```python
from build123d import *

# Parameters (mm, degrees)
SKETCH_1_R      = 4.5
SKETCH_1_R_2    = 2.5
EXTRUDE_1_DEPTH = 5
SKETCH_2_R      = 3
EXTRUDE_2_DEPTH = 28
EXTRUDE_3_DEPTH = 4
SKETCH_5_R      = 3
EXTRUDE_4_DEPTH = 5.5
EXTRUDE_6_DEPTH = 5
SKETCH_7_R      = 1.6
EXTRUDE_7_DEPTH = 1.4


with BuildPart() as part:
    # 草图1 → 凸台-拉伸1 (new body)
    with BuildSketch(Plane(origin=(0, 0, 0), x_dir=(0, 0, -1), z_dir=(1, 0, 0))):
        with BuildLine():
            Line((31.1, -15.85), (-21.1, -15.85))
            ThreePointArc((-21.1, -15.85), (-28.171067812, -12.921067812), (-31.1, -5.85))
            Line((-31.1, -5.85), (-31.1, 5.85))
            ThreePointArc((-31.1, 5.85), (-28.171067812, 12.921067812), (-21.1, 15.85))
            Line((-21.1, 15.85), (31.1, 15.85))
            Line((31.1, 15.85), (31.1, -15.85))
        make_face()
        with Locations((-11.1, 0)):
            Circle(SKETCH_1_R, mode=Mode.SUBTRACT)
        with Locations((13.4, 0)):
            Circle(SKETCH_1_R_2, mode=Mode.SUBTRACT)
    extrude(amount=EXTRUDE_1_DEPTH)

    # 草图2 → 凸台-拉伸2 (add)
    with BuildSketch(Plane(origin=(5, 0, 0), x_dir=(0, 0, -1), z_dir=(1, 0, 0))):
        with Locations((-28.1, 0)):
            Circle(SKETCH_2_R)
        with Locations((4.1, 11.85)):
            Circle(SKETCH_2_R)
        with Locations((4.1, -11.85)):
            Circle(SKETCH_2_R)
    extrude(amount=EXTRUDE_2_DEPTH)

    # 草图3 → 凸台-拉伸3 (add)
    with BuildSketch(Plane(origin=(33, 0, 0), x_dir=(0, 0, -1), z_dir=(1, 0, 0))):
        with BuildLine():
            Line((8.9, 15.85), (-21.1, 15.85))
            ThreePointArc((-21.1, 15.85), (-28.171067812, 12.921067812), (-31.1, 5.85))
            Line((-31.1, 5.85), (-31.1, 0))
            Line((-31.1, 0), (-31.1, -5.85))
            ThreePointArc((-31.1, -5.85), (-28.171067812, -12.921067812), (-21.1, -15.85))
            Line((-21.1, -15.85), (8.9, -15.85))
            Line((8.9, -15.85), (8.9, 15.85))
        make_face()
    extrude(amount=EXTRUDE_3_DEPTH)

    # 草图5 → 凸台-拉伸4 (add)
    with BuildSketch(Plane.ZY):
        with Locations((-27.1, 11.85)):
            Circle(SKETCH_5_R)
        with Locations((-27.1, -11.978090594)):
            Circle(SKETCH_5_R)
        with Locations((13.9, 11.85)):
            Circle(SKETCH_5_R)
        with Locations((13.9, -11.978090594)):
            Circle(SKETCH_5_R)
    extrude(amount=EXTRUDE_4_DEPTH)

    # 草图6 → 凸台-拉伸6 (add)
    with BuildSketch(Plane.ZY.offset(5.5)):
        with BuildLine():
            Line((15.255672946, -15.85), (-31.1, -15.85))
            Line((-31.1, -15.85), (-31.1, 15.85))
            Line((-31.1, 15.85), (15.255672946, 15.85))
            ThreePointArc((15.255672946, 15.85), (17.376993289, 14.971320344), (18.255672946, 12.85))
            Line((18.255672946, 12.85), (18.255672946, 9.183659284))
            ThreePointArc((18.255672946, 9.183659284), (17.376993289, 7.062338941), (15.255672946, 6.183659284))
            Line((15.255672946, 6.183659284), (8.696116264, 6.183659284))
            ThreePointArc((8.696116264, 6.183659284), (6.574795921, 5.304979628), (5.696116264, 3.183659284))
            Line((5.696116264, 3.183659284), (5.696116264, -3.183659284))
            ThreePointArc((5.696116264, -3.183659284), (6.574795921, -5.304979628), (8.696116264, -6.183659284))
            Line((8.696116264, -6.183659284), (15.255672946, -6.183659284))
            ThreePointArc((15.255672946, -6.183659284), (17.376993289, -7.062338941), (18.255672946, -9.183659284))
            Line((18.255672946, -9.183659284), (18.255672946, -12.85))
            ThreePointArc((18.255672946, -12.85), (17.376993289, -14.971320344), (15.255672946, -15.85))
        make_face()
    extrude(amount=EXTRUDE_6_DEPTH)

    # 草图7 → 凸台-拉伸7 (add)
    with BuildSketch(Plane.XZ.offset(15.85)):
        with Locations((2.5, 10.7)):
            Circle(SKETCH_7_R)
        with Locations((2.5, -23.1)):
            Circle(SKETCH_7_R)
    extrude(amount=EXTRUDE_7_DEPTH)


solid = part.part
```
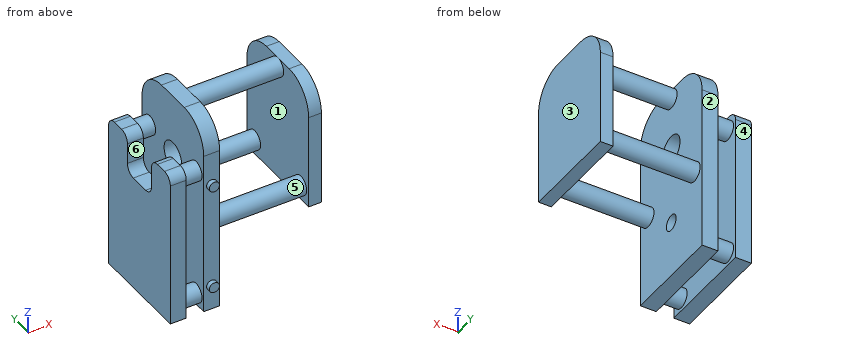
Here's how the part is built. I have some questions about the finished solid (model axes, mm). Face numbers are marked on the shaded views. A direction names the side the tool comes from. Coordinates: 2 decimals unless noted, no trailing zeros. Order: outer loops, then holes, each group sorted by start corner. A loop starts at its lowest first (then second) coordinate and runs counter-clockwise, first axis right, second up. Notation, with made-up numbers: (-26.5, 84) - (10.5, 84) arc R21 ccw to (10.5, 119) - close; hole circle Ø6 at (49.5, 66). An arc over 180 degrees is marked (long way). One line per question, with ' | ' between items.
(1) If I drill on L1, parallel to X at y = 9.5, z = 8; L2, parallel to X at y = -9.5, z = 22.5; L3, parallel to Y at x = 2, z = 11, over which ranges is the centre line in solid material (lowest first)?
Report:
L1: x = -10.5 to -5.5, 0 to 5, 33 to 37 | L2: x = 0 to 5, 33 to 37 | L3: y = -17.25 to -4.5, 4.5 to 15.85
(2) Suppose I cut it at B-B on z = -23.1. List the corners of the cut face in (x, y) for me.
Report:
outline: (-10.5, -15.85) - (-5.5, -15.85) - (-5.5, 15.85) - (-10.5, 15.85) - close; (0, -15.85) - (0.9, -15.85) - (0.9, -17.25) - (4.1, -17.25) - (4.1, -15.85) - (5, -15.85) - (5, 15.85) - (0, 15.85) - close
(3) For the marked faces 1 and 2, which set-ups out of +Z, -Z, +X, -X, +Y, -Y let a thin tool reach every point of the face, with its end or its side?
Report:
face 1: none | face 2: +Z, -Z, +X, -X, +Y
(4) Suppose I cut it at C-C on x = 2.5. List the corners of the cut face in (y, z) for me.
Report:
outline: (-17.25, -24.7) - (-15.85, -24.7) - (-15.85, -31.1) - (15.85, -31.1) - (15.85, 21.1) arc R10 ccw to (5.85, 31.1) - (-5.85, 31.1) arc R10 ccw to (-15.85, 21.1) - (-15.85, 12.3) - (-17.25, 12.3) - (-17.25, 9.1) - (-15.85, 9.1) - (-15.85, -21.5) - (-17.25, -21.5) - close; hole circle Ø9 at (0, 11.1); hole circle Ø5 at (0, -13.4)
(5) Suppose I cut it at A-A on z = -4.1. List the corners of the cut face in (x, y) for me, and give its area (3 significant figures).
Report:
outline: (-10.5, -15.85) - (-5.5, -15.85) - (-5.5, 15.85) - (-10.5, 15.85) - close; (0, -15.85) - (5, -15.85) - (5, -14.85) - (33, -14.85) - (33, -15.85) - (37, -15.85) - (37, 15.85) - (33, 15.85) - (33, 14.85) - (5, 14.85) - (5, 15.85) - (0, 15.85) - close; hole (5, -8.85) - (33, -8.85) - (33, 8.85) - (5, 8.85) - close | area: 780 mm2
(6) Will these pins go through, and if not, where does the flat tip stop? pin 1 (1.5 mm diameter, centred on x = -3, y = 2.5, fed in from +Z); pin 2 (3 mm diameter, centred on x = -7.5, y = 11, fed in from +Z); pin 3 (3 mm diameter, centred on y = 0, z = -13.4, fed in from +X); pin 4 (11.5 mm diameter, centred on y = 0, z = 11.1, fed in from -X).
Report:
pin 1: passes through | pin 2: stops at z = 18.26 | pin 3: stops at x = -5.5 | pin 4: stops at x = -10.5
(7) Suppose I cut it at D-D on x = 16. List the corners of the cut face in (y, z) for me, and give its area (3 significant figures).
Report:
outline: circle Ø6 at (-11.85, -4.1); circle Ø6 at (0, 28.1); circle Ø6 at (11.85, -4.1) | area: 84.8 mm2
(8) If we mould it in two halves opening along Y, with no side actions, what happens to the marked faces 3, 4, 5 and 6? For each: pulls with the +Y half, pulls with the -Y half, needs draft (parallel to the pull), parting line crosses it, or undercut.
Report:
face 3: needs draft | face 4: pulls with the +Y half | face 5: undercut | face 6: undercut
